Read the model definition and answer for the solid it produces. Units are mm, in the model's axes. A direction names the side the tool comes from. Coordinates: 2 decimals unless noted, no trailing zeros. Order: outer loops, then holes, each group sorted by start corner. A loop starts at its lowest first (then second) coordinate and runs counter-clockwise, first axis right, second up.
```python
from build123d import *

# Parameters (mm, degrees)
SKETCH2_W            = 109
SKETCH2_H            = 6
BOSS_EXTRUDE2_DEPTH  = 54
BOSS_EXTRUDE18_DEPTH = 3
BOSS_EXTRUDE14_DEPTH = 14.15
CUT_EXTRUDE7_DEPTH   = 23
CUT_EXTRUDE8_DEPTH   = 3
SKETCH33_W           = 6
SKETCH33_H           = 3
CUT_EXTRUDE9_DEPTH   = 123
SKETCH34_W           = 4
SKETCH34_H           = 4
CUT_EXTRUDE10_DEPTH  = 86


with BuildPart() as part:
    # Sketch2 → Boss-Extrude2 (new body)
    with BuildSketch(Plane(origin=(0, 0, 0), x_dir=(1, 0, 0), z_dir=(0, 1, 0))):
        with Locations((0, -61.5)):
            Rectangle(SKETCH2_W, SKETCH2_H)
    extrude(amount=BOSS_EXTRUDE2_DEPTH)

    # Sketch30 → Boss-Extrude18 (add)
    with BuildSketch(Plane(origin=(0, 0, 58.5), x_dir=(-1, 0, 0), z_dir=(0, 0, -1))):
        with BuildLine():
            Line((44.898046307, 54), (-54.5, 54))
            Line((-54.5, 54), (-54.5, 3))
            Line((-54.5, 3), (13.717264207, 3))
            Line((13.717264207, 3), (-4.931615029, 5.361896936))
            ThreePointArc((-4.931615029, 5.361896936), (-14.898890302, 10.119374153), (-20.065130462, 19.881040427))
            Line((-20.065130462, 19.881040427), (-23.157396088, 38.179135111))
            ThreePointArc((-23.157396088, 38.179135111), (-22.149967828, 41.451692308), (-18.921946876, 42.593805718))
            Line((-18.921946876, 42.593805718), (-0.511473267, 40.262103064))
            ThreePointArc((-0.511473267, 40.262103064), (9.455802006, 35.504625847), (14.622042166, 25.742959573))
            Line((14.622042166, 25.742959573), (18.46546266, 3))
            Line((18.46546266, 3), (26.071580329, 3))
            Line((26.071580329, 3), (20.034760857, 23.540167479))
            ThreePointArc((20.034760857, 23.540167479), (20.404648352, 34.578434964), (27.282125622, 43.220221367))
            Line((27.282125622, 43.220221367), (42.812477849, 53.378495603))
            ThreePointArc((42.812477849, 53.378495603), (43.809944346, 53.841319504), (44.898046307, 54))
        make_face()
        with BuildLine():
            Line((54.5, 3), (54.5, 25.946731257))
            Line((54.5, 25.946731257), (54.311662737, 25.932891577))
            ThreePointArc((54.311662737, 25.932891577), (51.728512948, 19.022816741), (46.538874378, 13.779778633))
            Line((46.538874378, 13.779778633), (30.058342822, 3))
            Line((30.058342822, 3), (54.5, 3))
        make_face()
    extrude(amount=BOSS_EXTRUDE18_DEPTH)

    # Sketch26 → Boss-Extrude14 (add)
    with BuildSketch(Plane(origin=(0, 0, 58.5), x_dir=(-1, 0, 0), z_dir=(0, 0, -1))):
        with BuildLine():
            Line((-32.835842822, 3), (-28.849080329, 3))
            Line((-28.849080329, 3), (-22.812260857, 23.540167479))
            ThreePointArc((-22.812260857, 23.540167479), (-23.182148352, 34.578434964), (-30.059625622, 43.220221367))
            Line((-30.059625622, 43.220221367), (-45.589977849, 53.378495603))
            ThreePointArc((-45.589977849, 53.378495603), (-48.161514659, 53.968880093), (-50.5, 52.747061074))
            Line((-50.5, 52.747061074), (-50.5, 14.625881424))
            ThreePointArc((-50.5, 14.625881424), (-49.916939273, 14.190586609), (-49.316374378, 13.779778633))
            Line((-49.316374378, 13.779778633), (-32.835842822, 3))
        make_face()
    extrude(amount=BOSS_EXTRUDE14_DEPTH)

    # Sketch9 → Cut-Extrude7 (cut)
    with BuildSketch(Plane.XY.offset(64.5)):
        with BuildLine():
            ThreePointArc((-42.752881471, 50.979977107), (-45.688023414, 52.335164835), (-47.043211142, 49.400022893))
            ThreePointArc((-47.043211142, 49.400022893), (-44.108069199, 48.044835165), (-42.752881471, 50.979977107))
        make_face()
        with BuildLine():
            ThreePointArc((-31.068118529, 6.020022893), (-28.132976586, 4.664835165), (-26.777788858, 7.599977107))
            ThreePointArc((-26.777788858, 7.599977107), (-29.712930801, 8.955164835), (-31.068118529, 6.020022893))
        make_face()
        with BuildLine():
            ThreePointArc((-15.540189678, 8.459583143), (-15.607157436, 5.227384615), (-12.374958909, 5.160416857))
            ThreePointArc((-12.374958909, 5.160416857), (-12.307991151, 8.392615385), (-15.540189678, 8.459583143))
        make_face()
        with BuildLine():
            ThreePointArc((20.983277975, 37.164416857), (21.050245733, 40.396615385), (17.818047205, 40.463583143))
            ThreePointArc((17.818047205, 40.463583143), (17.751079447, 37.231384615), (20.983277975, 37.164416857))
        make_face()
        with BuildLine():
            ThreePointArc((29.555288858, 7.599977107), (30.910476586, 4.664835165), (33.845618529, 6.020022893))
            ThreePointArc((33.845618529, 6.020022893), (32.490430801, 8.955164835), (29.555288858, 7.599977107))
        make_face()
        with BuildLine():
            ThreePointArc((49.820711142, 49.400022893), (48.465523414, 52.335164835), (45.530381471, 50.979977107))
            ThreePointArc((45.530381471, 50.979977107), (46.885569199, 48.044835165), (49.820711142, 49.400022893))
        make_face()
    extrude(amount=-CUT_EXTRUDE7_DEPTH, mode=Mode.SUBTRACT)

    # Sketch24 → Cut-Extrude8 (cut)
    with BuildSketch(Plane.XY.offset(64.5)):
        Polygon((-40.856594422, 50.19), (-42.877320364, 53.69), (-46.918772249, 53.69), (-48.939498191, 50.19), (-46.918772249, 46.69), (-42.877320364, 46.69), align=None)
        Polygon((51.716998191, 50.19), (49.696272249, 53.69), (45.654820364, 53.69), (43.634094422, 50.19), (45.654820364, 46.69), (49.696272249, 46.69), align=None)
        Polygon((35.741905578, 6.81), (33.721179636, 10.31), (29.679727751, 10.31), (27.659001809, 6.81), (29.679727751, 3.31), (33.721179636, 3.31), align=None)
        Polygon((-9.916122409, 6.81), (-11.936848352, 10.31), (-15.978300236, 10.31), (-17.999026178, 6.81), (-15.978300236, 3.31), (-11.936848352, 3.31), align=None)
        Polygon((23.442114474, 38.814), (21.421388532, 42.314), (17.379936648, 42.314), (15.359210706, 38.814), (17.379936648, 35.314), (21.421388532, 35.314), align=None)
        Polygon((-24.881501809, 6.81), (-26.902227751, 10.31), (-30.943679636, 10.31), (-32.964405578, 6.81), (-30.943679636, 3.31), (-26.902227751, 3.31), align=None)
    extrude(amount=-CUT_EXTRUDE8_DEPTH, mode=Mode.SUBTRACT)

    # Sketch33 → Cut-Extrude9 (cut)
    with BuildSketch(Plane.ZY.offset(54.5)):
        with Locations((61.5, 1.5)):
            Rectangle(SKETCH33_W, SKETCH33_H)
    extrude(amount=-CUT_EXTRUDE9_DEPTH, mode=Mode.SUBTRACT)

    # Sketch34 → Cut-Extrude10 (cut)
    with BuildSketch(Plane(origin=(0, 54, 0), x_dir=(1, 0, 0), z_dir=(0, 1, 0))):
        with Locations((-52.5, -62.5)):
            Rectangle(SKETCH34_W, SKETCH34_H)
        with Locations((52.5, -62.5)):
            Rectangle(SKETCH34_W, SKETCH34_H)
    extrude(amount=-CUT_EXTRUDE10_DEPTH, mode=Mode.SUBTRACT)


solid = part.part
```
1) Flat-ended cylindrical pins translate along their axes: pin 1 Ø4 at (y, z) = (14.5, 48) entering from -X; pin 2 Ø5 at (x, z) = (24, 47.5) entering from +Y; pin 3 Ø3 at (y, z) = (21.5, 62.5) entering from -X. Find the tip coordinate at first contact, or state that the pin passes through.
A:
pin 1: stops at x = 24.88
pin 2: stops at y = 40.14
pin 3: stops at x = -50.5
2) A cutting plane is placed at B-B, the plane z = 52.5. Determine the outline of the cut face in (x, y), and give its area (3 significant figures).
A:
outline: (22.81, 23.54) - (28.85, 3) - (32.84, 3) - (49.32, 13.78) arc R17.59 ccw to (50.5, 14.63) - (50.5, 52.75) arc R3.81 ccw to (45.59, 53.38) - (30.06, 43.22) arc R17.59 ccw to start; hole circle Ø4.57 at (31.7, 6.81); hole circle Ø4.57 at (47.68, 50.19)
area: 1,030 mm2
3) A cutting plane is placed at C-C, the plane x = -3. Determine the outline of the cut face in (y, z).
A:
outline: (3, 55.5) - (4.36, 55.5) - (4.36, 58.5) - (39.44, 58.5) - (39.44, 55.5) - (54, 55.5) - (54, 64.5) - (3, 64.5) - close
4) Which of the six approach directions +Z, -Z, +X, -X, +Y, -Y give full straight-line access (tool end or side, diameter ignored) to faces 1 (the flat face through (21.59, 28.9, 57.02)), 2 (the flat face through (20.2, 41.2, 61.5)), 3 (the cylindrical face through (-43.8, 53.84, 57.02))?
A:
face 1: -Z
face 2: +Z
face 3: -Z, -X
5) Straight lines are drawn through the part: line 1 (Z direction, x = -5, y = 24); line 2 (Y direction, x = 46, z = 60.25); line 3 (Z direction, x = -17, y = 28.5). For each, find the intervals that lie inside material, in ascending order.
A:
line 1: z = 58.5 to 64.5
line 2: y = 3 to 48.63, 51.75 to 54
line 3: z = 55.5 to 64.5
6) Determine the mould class of faces 4 (the flat face through (50.5, 34, 50)), 5 (the flat face through (44.63, 48.464, 63.021)), 6 (the flat face through (1, 3, 61)) for opening direction Y: pulls with the +Y half, pulls with the -Y half, needs draft (parallel to the pull), parting line crosses it, or undercut.
A:
face 4: needs draft
face 5: undercut
face 6: pulls with the -Y half
7) A cutting plane is placed at A-A, the plane z = 57.25. Determine the outline of the cut face in (x, y), and give its area (3 significant figures).
A:
outline: (-54.5, 3) - (-30.06, 3) - (-46.54, 13.78) arc R17.59 cw to (-54.31, 25.93) - (-54.5, 25.95) - close; (-44.9, 54) arc R3.81 cw to (-42.81, 53.38) - (-27.28, 43.22) arc R17.59 cw to (-20.03, 23.54) - (-26.07, 3) - (-18.47, 3) - (-14.62, 25.74) arc R17.59 cw to (0.51, 40.26) - (18.92, 42.59) arc R3.81 cw to (23.16, 38.18) - (20.07, 19.88) arc R17.59 cw to (4.93, 5.36) - (-13.72, 3) - (54.5, 3) - (54.5, 54) - close; hole circle Ø4.57 at (31.7, 6.81); hole circle Ø4.57 at (47.68, 50.19)
area: 3,010 mm2
